The listing builds one solid part. Answer for the finished solid, in the listing's coordinates (mm). A direction names the side the tool comes from. Round coordinates to 2 decimals unless told otherwise and drop trailing zeros. Write each loop counter-clockwise with the first axis right and the second up, starting at its lowest first coordinate (ties: lowest second). Pieces come first, ordered by that corner, then holes. Notation, with made-up numbers: (-12.75, 75) - (23.25, 75) arc R16 cw to (23.25, 93) - close; hole circle Ø9 at (3, 63.25). An arc over 180 degrees is marked (long way). Return JSON: item names as keys, results as strings. Group by question number.
(1) Find the intervals of material crossed by line 1 along Y through (x, z) = (0, 3); line 2 along Z through (x, y) = (6, 2.75); line 3 along Y through (x, z) = (-0.75, 2.8), in increasing order. Write a range as [from, to].
(2) Section C-C, the plane x = -7 is taken. Write down the section's boundary in (y, z).
(3) Determine the mould class of faces 1 (the conical face through (4.859, -2.617, 1.458)), 2 (the flat face through (3.5, 5, 3)), 3 (the flat face through (-1.8, 2, 2.7)), 4 (the cylindrical face through (-2.17, -9.76, 0.35)) for opening direction X: +X half, -X half, draft (parallel to the pull), parting line (faces both ways), or undercut.
(4) Each of these flat-tipped pins is pushed along its axis until it touches: pin 1 (4 mm diameter, centred on x = -1, y = -7, fed in from +Z); pin 2 (0.9 mm diameter, centred on y = 5.5, z = 2.5, fed in from -X); pin 3 (2 mm diameter, centred on y = -4.5, z = 3, fed in from -X). Where does it stop, or does it pass through?
(5) Section B-B, the plane y = 5 is taken. Write down the section's boundary in (x, z), then the cut area to 3 significant figures.
(6) Section A-A, the plane z = 2.3 is taken. Write down the section's boundary in (x, y) (3 decimals).
(7) Section D-D, the plane z = 3.7 is taken. Write down the section's boundary in (x, y) (3 decimals).
(8) Which of the six approach directions +Z, -Z, +X, -X, +Y, -Y give full straight-line access (tool end or side, diameter ignored) to faces 5 (the flat face through (1.728, 1.956, 2.679)), 6 (the flat face through (1.8, 8, 2.7)), 7 (the flat face through (0, 0, 0.7))?
```python
from build123d import *

# Parameters (mm, degrees)
SKETCH1_R           = 10
BOSS_EXTRUDE1_DEPTH = 0.7
REVOLVE1_ANGLE      = 180
SKETCH2_5_R         = 3.5
BOSS_EXTRUDE2_DEPTH = 5
BOSS_EXTRUDE2_TAPER = 45
BOSS_EXTRUDE3_DEPTH = 3.5
FILLET1_R           = 0.35
SKETCH3_R           = 2
CUT_EXTRUDE1_DEPTH  = 10
FILLET2_R           = 0.5


with BuildPart() as part:
    # Sketch1 → Boss-Extrude1 (new body)
    with BuildSketch(Plane.XY):
        Circle(SKETCH1_R)
    extrude(amount=BOSS_EXTRUDE1_DEPTH)

    # Sketch2 → Revolve1 (revolve)
    with BuildSketch(Plane.XY.offset(0.7)):
        with BuildLine():
            Line((-4.330127019, -6), (-4.330127019, 1))
            ThreePointArc((-4.330127019, 1), (-7.830127019, -2.5), (-4.330127019, -6))
        make_face()
    revolve(axis=Axis((-4.330127019, -6, 0.7), (0, 1, 0)), revolution_arc=REVOLVE1_ANGLE)

    # Sketch2<5> → Boss-Extrude2 (add)
    with BuildSketch(Plane.XY.offset(0.7)):
        with Locations((4.330127019, -2.5)):
            Circle(SKETCH2_5_R)
    extrude(amount=BOSS_EXTRUDE2_DEPTH, taper=BOSS_EXTRUDE2_TAPER)

    # Sketch2<6> → Boss-Extrude3 (add)
    with BuildSketch(Plane.XY.offset(0.7)):
        Polygon((0, 0.958548116), (3.5, 2.979274058), (3.5, 7.020725942), (0, 9.041451884), (-3.5, 7.020725942), (-3.5, 2.979274058), align=None)
    extrude(amount=BOSS_EXTRUDE3_DEPTH)

    # Fillet1
    fillet1_edges = [part.edges().sort_by_distance(p)[0] for p in [
        (-3.5, 7.020725942, 2.45),
        (-3.5, 2.979274058, 2.45),
        (0, 0.958548116, 2.45),
        (3.5, 2.979274058, 2.45),
        (3.5, 7.020725942, 2.45),
        (0, 9.041451884, 2.45),
    ]]
    fillet(fillet1_edges, radius=FILLET1_R)

    # Sketch3 → Cut-Extrude1 (cut)
    with BuildSketch(Plane.XY.offset(4.2)):
        with Locations((0, 5)):
            Circle(SKETCH3_R)
    extrude(amount=-CUT_EXTRUDE1_DEPTH, mode=Mode.SUBTRACT)

    # Fillet2
    fillet2_edges = [part.edges().sort_by_distance(p)[0] for p in [
        (-1.75, 8.031088913, 0.7),
        (1.75, 8.031088913, 0.7),
        (-3.5, 5, 0.7),
        (-1.75, 1.968911087, 0.7),
        (3.5, 5, 0.7),
        (1.75, 1.968911087, 0.7),
        (0, 8.987306696, 0.7),
        (-3.453108891, 6.993653348, 0.7),
        (-3.453108891, 3.006346652, 0.7),
        (3.453108891, 6.993653348, 0.7),
        (3.453108891, 3.006346652, 0.7),
        (0, 1.012693304, 0.7),
    ]]
    fillet(fillet2_edges, radius=FILLET2_R)

    # Cut-Extrude2 cone 1 section (through the dimple's axis) → Cut-Extrude2 (revolve, cut)
    with BuildSketch(Plane(origin=(4.330127019, -2.5, 0), x_dir=(0, 1, 0), z_dir=(1, 0, 0))):
        Polygon((0, 0), (2, 0), (0, 2), align=None)
    revolve(axis=Axis((4.330127019, -2.5, 0), (0, 0, 1)), mode=Mode.SUBTRACT)


solid = part.part
```
Working result:
{
 "1": {"line 1": "y = [1.01, 3], [7, 8.99]", "line 2": "z = [0, 0.7]", "line 3": "y = [1.39, 3.15], [6.85, 8.61]"},
 "2": {"outline": "(-7.14, 0) - (7.14, 0) - (7.14, 0.7) - (-0.24, 0.7) arc R2.26 ccw to (-4.76, 0.7) - (-7.14, 0.7) - close"},
 "3": {"face 1": "undercut", "face 2": "+X half", "face 3": "-X half", "face 4": "parting line"},
 "4": {"pin 1": "stops at z = 0.7", "pin 2": "stops at x = -3.5", "pin 3": "stops at x = -7.17"},
 "5": {"outline": "(-8.66, 0) - (-2, 0) - (-2, 4.2) - (-3.5, 4.2) - (-3.5, 1.2) arc R0.5 cw to (-4, 0.7) - (-8.66, 0.7) - close; (2, 0) - (8.66, 0) - (8.66, 0.7) - (4, 0.7) arc R0.5 cw to (3.5, 1.2) - (3.5, 4.2) - (2, 4.2) - close", "area": "19.9 mm^2"},
 "6": {"outline": "circle Ø6.226 at (-4.33, -2.5); (-3.5, 3.181) arc R0.35 ccw to (-3.325, 2.878) - (-0.175, 1.06) arc R0.35 ccw to (0.175, 1.06) - (3.325, 2.878) arc R0.35 ccw to (3.5, 3.181) - (3.5, 6.819) arc R0.35 ccw to (3.325, 7.122) - (0.175, 8.94) arc R0.35 ccw to (-0.175, 8.94) - (-3.325, 7.122) arc R0.35 ccw to (-3.5, 6.819) - close; circle Ø3.8 at (4.33, -2.5); hole circle Ø4 at (0, 5)"},
 "7": {"outline": "circle Ø3.606 at (-4.33, -2.5); (-3.5, 3.181) arc R0.35 ccw to (-3.325, 2.878) - (-0.175, 1.06) arc R0.35 ccw to (0.175, 1.06) - (3.325, 2.878) arc R0.35 ccw to (3.5, 3.181) - (3.5, 6.819) arc R0.35 ccw to (3.325, 7.122) - (0.175, 8.94) arc R0.35 ccw to (-0.175, 8.94) - (-3.325, 7.122) arc R0.35 ccw to (-3.5, 6.819) - close; circle Ø1 at (4.33, -2.5); hole circle Ø4 at (0, 5)"},
 "8": {"face 5": "+Z, +X", "face 6": "+Z, +X, +Y", "face 7": "+Z"}
}
